from build123d import *

# Parameters (mm, degrees)
F0_W      = 170
F0_H      = 100
F1_DEPTH  = 2
F2_W      = 170
F2_H      = 100
F3_DEPTH  = 26
F4_W      = 2
F4_H      = 96
F5_DEPTH  = 26
F6_W      = 14
F6_H      = 96
F7_DEPTH  = 30
F8_W      = 10
F8_H      = 2.5
F9_DEPTH  = 10
F11_DEPTH = 26
F13_DEPTH = 30
F14_R     = 0.5


with BuildPart() as f1:
    # F0 (on Top) → F1 (new body)
    with BuildSketch(Plane.XY):
        with Locations((0.7212153077, -50)):
            Rectangle(F0_W, F0_H)
    extrude(amount=F1_DEPTH)

    # F2 (on face) → F3 (join)
    with BuildSketch(Plane.XY.offset(2)):
        with Locations((0.7212153077, -50)):
            Rectangle(F2_W, F2_H)
        Polygon((83.7212153077, -2), (83.7212153077, -98), (-82.2787846923, -98), (-82.8941488059, -2), align=None, mode=Mode.SUBTRACT)
    extrude(amount=F3_DEPTH)

    # F4 (on face) → F5 (join)
    with BuildSketch(Plane.XY.offset(2)):
        with Locations((68.7212153077, -50)):
            Rectangle(F4_W, F4_H)
    extrude(amount=F5_DEPTH)

    # F6 (on face) → F7 (cut)
    with BuildSketch(Plane.XY.offset(28)):
        with Locations((76.7212153077, -50)):
            Rectangle(F6_W, F6_H)
        Polygon((83.7212153077, -98), (69.7212153077, -98), (69.7212153077, -100), (85.7212153077, -100), (85.7212153077, 0), (69.7212153077, 0), (69.7212153077, -2), (83.7212153077, -2), align=None)
    extrude(amount=-F7_DEPTH, mode=Mode.SUBTRACT)

    # F8 (on face) → F9 (join)
    with BuildSketch(Plane.XZ.offset(100)):
        with Locations((-2.2787846923, 15.25)):
            Rectangle(F8_W, F8_H)
        with Locations((-12.2787846923, 15.25)):
            Rectangle(F8_W, F8_H)
        with Locations((-12.2787846923, 12.75)):
            Rectangle(F8_W, F8_H)
        with Locations((-2.2787846923, 12.75)):
            Rectangle(F8_W, F8_H)
    extrude(amount=F9_DEPTH)

    # F10 (on face) → F11 (join)
    with BuildSketch(Plane.XY.offset(2)):
        Polygon((67.7212153077, -15.9997123883), (-82.8044100496, -15.9997123883), (-82.7915902273, -17.9996713009), (67.7212153077, -17.9996713009), align=None)
    extrude(amount=F11_DEPTH)

    # F12 (on face) → F13 (cut)
    with BuildSketch(Plane.XY.offset(28)):
        Polygon((-84.2787846923, -15.9997123883), (-82.8044100496, -15.9997123883), (-82.8941488059, -2), (67.7212153077, -2), (67.7212153077, -15.9997123883), (69.7212153077, -15.9997123883), (69.7212153077, 0), (-84.2787846923, 0), align=None)
        Polygon((-82.8941488059, -2), (-82.8044100496, -15.9997123883), (67.7212153077, -15.9997123883), (67.7212153077, -2), align=None)
    extrude(amount=-F13_DEPTH, mode=Mode.SUBTRACT)

    # F14
    f14_edges = [f1.edges().sort_by_distance(p)[0] for p in [
        (-82.535187, -57.999836, 28),
        (-7.535187, -17.999671, 28),
        (-7.278785, -15.999712, 28),
        (-84.278785, -57.999856, 28),
        (-7.278785, -98, 28),
        (-7.278785, -100, 28),
        (67.721215, -57.999836, 28),
        (69.721215, -57.999856, 28),
        (69.721215, -15.999712, 14),
        (69.721215, -100, 14),
        (2.721215, -105, 16.5),
        (2.721215, -105, 11.5),
        (2.721215, -100, 14),
        (-7.278785, -100, 16.5),
        (-7.278785, -110, 16.5),
        (-7.278785, -110, 11.5),
        (-17.278785, -110, 14),
        (-84.278785, -100, 14),
        (-84.278785, -15.999712, 14),
        (-17.278785, -100, 14),
        (-17.278785, -105, 11.5),
        (2.721215, -110, 14),
        (-7.278785, -100, 11.5),
    ]]
    fillet(f14_edges, radius=F14_R)


solid = f1.part
Input: part model. Units: mm. Frame: model coordinates. A direction names the side the tool comes from. Coordinates: 2 decimals unless noted, no trailing zeros. Write each loop counter-clockwise with the first axis right and the second up, starting at its lowest first coordinate (ties: lowest second). Pieces come first, ordered by that corner, then holes. Notation, with made-up numbers: M 89,-33 L 138,-33 A22 ccw 138,-14 Z; hole C 18,2 d4. An arc over 180 degrees is marked long. Answer as a JSON object with one key per item and string values. Group by question number.
(1) Section A-A on z = 23. Output: boundary loops of the cut face in (x, y), plus the area to 3 significant figures.
(2) Set-up query: faces 1 (the face through (-6, -98, 15)), 2 (the face through (-17.279, -105, 14)), 3 (the face through (2.721, -105, 14)). Return all of +Z, -Z, +X, -X, +Y, -Y with unobstructed straight access to the full face (end or side cutting, diameter ignored); none if empty.
(3) Section C-C on x = -24. Output: boundary loops of the cut face in (y, z), plus the area to 3 significant figures.
(4) Section B-B on x = -4.5. Output: boundary loops of the cut face in (y, z), plus the area to 3 significant figures.
(5) Ray query, line 1 along Y through (x, z) = (-64, 19); line 2 along Z through (x, y) = (-57, -45); line 3 along X through (y, z) = (-23, 16.25). Return the intervals inside material, ascending. Write a range as [from, to].
(6) Contact query for flat-ended pins moving along their axis: P1, Ø6, axis at x = -20, y = -59, coming from the +Z side; P2, Ø5, axis at y = -106, z = 15, coming from the -X side; P3, Ø13, axis at x = 23, z = 18, coming from the -Y side. Output: stop coordinate, or through.
Result set:
{
 "1": {"outline": "M -84.28,-99.5 A0.5 ccw -83.78,-100 L 69.22,-100 A0.5 ccw 69.72,-99.5 L 69.72,-16.5 A0.5 ccw 69.22,-16 L -83.78,-16 A0.5 ccw -84.28,-16.5 Z; hole M -82.79,-18 L -82.28,-98 L 67.72,-98 L 67.72,-18 Z", "area": "915 mm2"},
 "2": {"face 1": "+Z", "face 2": "+Z, -Z, -X, -Y", "face 3": "+Z, -Z, +X, -Y"},
 "3": {"outline": "M -100,0 L -16,0 L -16,27.5 A0.5 ccw -16.5,28 L -17.5,28 A0.5 ccw -18,27.5 L -18,2 L -98,2 L -98,27.5 A0.5 ccw -98.5,28 L -99.5,28 A0.5 ccw -100,27.5 Z", "area": "272 mm2"},
 "4": {"outline": "M -110,12 A0.5 ccw -109.5,11.5 L -100.5,11.5 A0.5 cw -100,11 L -100,0 L -16,0 L -16,27.5 A0.5 ccw -16.5,28 L -17.5,28 A0.5 ccw -18,27.5 L -18,2 L -98,2 L -98,27.5 A0.5 ccw -98.5,28 L -99.5,28 A0.5 ccw -100,27.5 L -100,17 A0.5 cw -100.5,16.5 L -109.5,16.5 A0.5 ccw -110,16 Z", "area": "322 mm2"},
 "5": {"line 1": "y = [-100, -98], [-18, -16]", "line 2": "z = [0, 2]", "line 3": "x = [-84.28, -82.76], [67.72, 69.72]"},
 "6": {"P1": "stops at z = 2", "P2": "stops at x = -17.28", "P3": "stops at y = -100"}
}
